```python
from build123d import *

# Parameters (mm, degrees)
SKETCH_1_R          = 12
EXTRUDE_1_DEPTH     = 54.3
SKETCH_2_R          = 3.4
SKETCH_2_R_2        = 1.95
EXTRUDE_2_DEPTH     = 2.6
SKETCH_3_R          = 1.95
EXTRUDE_3_DEPTH     = 12
CUT_EXTRUDE_START   = -8
CUT_EXTRUDE_1_DEPTH = 8


with BuildPart() as part:
    # 草图1 → 凸台-拉伸1 (new body)
    with BuildSketch(Plane(origin=(0, 0, 0), x_dir=(1, 0, 0), z_dir=(0, 1, 0))):
        with Locations(Location((0, 0, 0), (0, 0, 90))):
            Circle(SKETCH_1_R)
    extrude(amount=EXTRUDE_1_DEPTH)

    # 草图2 → 凸台-拉伸2 (add)
    with BuildSketch(Plane(origin=(0, 54.3, 0), x_dir=(1, 0, 0), z_dir=(0, 1, 0))):
        with Locations(Location((0, 0, 0), (0, 0, 270))):
            Circle(SKETCH_2_R)
        with Locations(Location((0, 0, 0), (0, 0, 270))):
            Circle(SKETCH_2_R_2, mode=Mode.SUBTRACT)
    extrude(amount=EXTRUDE_2_DEPTH)

    # 草图3 → 凸台-拉伸3 (add)
    with BuildSketch(Plane(origin=(0, 54.3, 0), x_dir=(1, 0, 0), z_dir=(0, 1, 0))):
        with Locations(Location((0, 0, 0), (0, 0, 270))):
            Circle(SKETCH_3_R)
    extrude(amount=EXTRUDE_3_DEPTH)

    # 草图4 → 切除-拉伸1 (cut)
    with BuildSketch(Plane(origin=(0, 66.3, 0), x_dir=(1, 0, 0), z_dir=(0, 1, 0)).offset(CUT_EXTRUDE_START)):
        with BuildLine():
            Line((-1.5, 1.245993579), (1.5, 1.245993579))
            ThreePointArc((1.5, 1.245993579), (0, 1.95), (-1.5, 1.245993579))
        make_face()
    extrude(amount=CUT_EXTRUDE_1_DEPTH, mode=Mode.SUBTRACT)

    # 草图5 → 切除-旋转1 (revolve, cut)
    with BuildSketch(Plane(origin=(0, 0, 0), x_dir=(0, 0, -1), z_dir=(1, 0, 0))):
        Polygon((12, 31.3), (11, 31.3), (11, 30.7), (11.7, 30.7), (11.7, 0), (12, 0), (12, 30.7), align=None)
    revolve(axis=Axis((0, -3.315, 0), (0, 1, 0)), mode=Mode.SUBTRACT)


solid = part.part
```
Can you work these out from the model? Positions are in its coordinate system, mm. A direction names the side the tool comes from. Round coordinates to 2 decimals unless told otherwise and drop trailing zeros. Order: outer loops, then holes, each group sorted by start corner. A loop starts at its lowest first (then second) coordinate and runs counter-clockwise, first axis right, second up. Notation, with made-up numbers: (-20, 25.25) -> (-1, 25.25) arc R23 cw to (-1, 42.25) -> close; hole circle Ø2 at (87, 39). An arc over 180 degrees is marked (long way). Return JSON: item names as keys, results as strings. Group by question number.
1. If we section it at A-A, the plane z = 0: Write out the boundary of the cut face in (x, y), then the cut area to 3 significant figures.
2. Which directions (+Z, -Z, +X, -X, +Y, -Y) give clear straight access to the entire face, cutting with the end or side of a thin tool? Please do faces 1 (the face through (11.42, 15.14, 2.54)), 2 (the face through (0, 62, -1.246)), 3 (the face through (10, 31.3, -5)), 4 (the face through (-1.5, 56.9, 1.5)).
3. I need wall thicknesses on line 1 (Y direction, x = 1, z = -11); line 2 (Y direction, x = 1.75, z = 3.25); line 3 (Y direction, x = -2, z = -0.5). Which ranges of each line are inside material? Lowest first, please. Write a range as [from, to].
4. If we section it at C-C, the plane y = 40: Write out the boundary of the cut face in (x, z), then the cut area to 3 significant figures.
5. If we section it at B-B, the plane x = 0: Write out the boundary of the cut face in (y, z).
6. Will these pins go through, and if not, where does the flat tip stop? pin 1 (1 mm diameter, centred on y = 15.5, z = 7.5, fed in from -X); pin 2 (0.8 mm diameter, centred on x = -0.5, z = -2, fed in from +Y); pin 3 (1.5 mm diameter, centred on x = -0.5, y = 61.5, fed in from -Z); pin 4 (12 mm diameter, centred on x = 3, y = 48.5, fed in from +Z).
7. We'd pull the mould along Y, two halves only. Please class faces 5 (the face through (10.74, 31, 2.38)), 6 (the face through (0, 66.3, 0)), 7 (the face through (-3.604, 42.639, -11.446)), 8 (the face through (7, 30.7, 9)): released by +Y, released by -Y, zero draft, split by the parting line, or undercut.
8. If we section it at D-D, the plane z = -10: Write out the boundary of the cut face in (x, y), then the cut area to 3 significant figures.
Output values:
{
 "1": {"outline": "(-12, 31.3) -> (-11, 31.3) -> (-11, 30.7) -> (-11.7, 30.7) -> (-11.7, 0) -> (11.7, 0) -> (11.7, 30.7) -> (11, 30.7) -> (11, 31.3) -> (12, 31.3) -> (12, 54.3) -> (3.4, 54.3) -> (3.4, 56.9) -> (1.95, 56.9) -> (1.95, 66.3) -> (-1.95, 66.3) -> (-1.95, 56.9) -> (-3.4, 56.9) -> (-3.4, 54.3) -> (-12, 54.3) -> close", "area": "1,340 mm²"},
 "2": {"face 1": "-Y", "face 2": "-Z, +X, -X, +Y", "face 3": "none", "face 4": "+Y"},
 "3": {"line 1": "[0, 30.7], [31.3, 54.3]", "line 2": "[0, 54.3]", "line 3": "[0, 56.9]"},
 "4": {"outline": "circle Ø24 at (0, 0)", "area": "452 mm²"},
 "5": {"outline": "(0, -11.7) -> (30.7, -11.7) -> (30.7, -11) -> (31.3, -11) -> (31.3, -12) -> (54.3, -12) -> (54.3, -3.4) -> (56.9, -3.4) -> (56.9, -1.95) -> (58.3, -1.95) -> (58.3, -1.25) -> (66.3, -1.25) -> (66.3, 1.95) -> (56.9, 1.95) -> (56.9, 3.4) -> (54.3, 3.4) -> (54.3, 12) -> (31.3, 12) -> (31.3, 11) -> (30.7, 11) -> (30.7, 11.7) -> (0, 11.7) -> close"},
 "6": {"pin 1": "x = -9.37", "pin 2": "y = 58.3", "pin 3": "z = -1.25", "pin 4": "z = 12"},
 "7": {"face 5": "undercut", "face 6": "released by +Y", "face 7": "zero draft", "face 8": "undercut"},
 "8": {"outline": "(-6.63, 31.3) -> (-4.58, 31.3) -> (-4.58, 30.7) -> (-6.07, 30.7) -> (-6.07, 0) -> (6.07, 0) -> (6.07, 30.7) -> (4.58, 30.7) -> (4.58, 31.3) -> (6.63, 31.3) -> (6.63, 54.3) -> (-6.63, 54.3) -> close", "area": "684 mm²"}
}
